Read the model definition and answer for the solid it produces. Units are mm, in the model's axes. Face numbers are marked on the shaded views. A direction names the side the tool comes from. Round coordinates to 2 decimals unless told otherwise and drop trailing zeros. Order: outer loops, then holes, each group sorted by start corner. A loop starts at its lowest first (then second) coordinate and runs counter-clockwise, first axis right, second up. Notation, with made-up numbers: (10.5, -15) -> (22.5, -15) arc R4 cw to (22.5, -8) -> close; hole circle Ø5 at (32, 24). An arc over 180 degrees is marked (long way). Use a Markdown table: item, result. Add a question column.
1. The mould has two halves that part along Z. Classify the marked faces 1, 2, 3 and 4: +Z half, -Z half, draft (parallel to the pull), parting line (faces both ways), or undercut.
2. Given pin 1 (8 mm diameter, centred on x = -3.5, z = 22, fed in from -Y), flat-ended and moving along its own axis, determine where the tip first touches the part or whether it passes through.
3. For the marked faces 5 and 6, determine the directions among +Z, -Z, +X, -X, +Y, -Y from which every point of the face is accessible in a straight line to the end or side of a thin tool.
4. Section A-A, the plane x = 0 is taken. Give the vertices of the cut face in (y, z).
5. Section B-B, the plane z = 1 is taken. Give the vertices of the cut face in (x, y), then the cut area to 3 significant figures.
6. Section C-C, the plane y = 1.75 is taken. Give the vertices of the cut face in (x, z), then the cut area to 3 significant figures.
7. Consider L1, parallel to Z at x = -0.5, y = 5.25; L2, parallel to Z at x = -10, y = -3.25; L3, parallel to X at y = -1, z = 4. Determine where each line is inside the solid, lowest interval first. Write a range as [from, to].
8. Section D-D, the plane z = 18.5 is taken. Give the vertices of the cut face in (x, y).
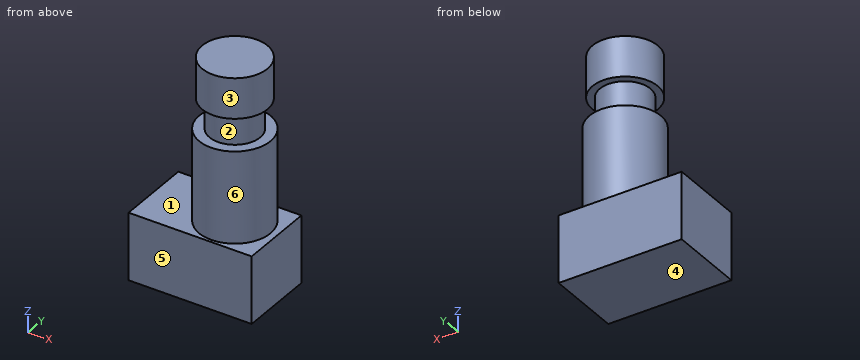
```python
from build123d import *

# Parameters (mm, degrees)
CROQUIS1_R              = 5.85
SALIENTE_EXTRUIR1_DEPTH = 15
CROQUIS2_R              = 4.15
SALIENTE_EXTRUIR2_DEPTH = 5
CROQUIS3_R              = 5.35
SALIENTE_EXTRUIR3_DEPTH = 6.6
CROQUIS4_W              = 20.15
CROQUIS4_H              = 12.4
SALIENTE_EXTRUIR4_DEPTH = 11


with BuildPart() as part:
    # Croquis1 → Saliente-Extruir1 (new body)
    with BuildSketch(Plane.XY):
        Circle(CROQUIS1_R)
    extrude(amount=SALIENTE_EXTRUIR1_DEPTH)

    # Croquis2 → Saliente-Extruir2 (add)
    with BuildSketch(Plane.XY.offset(15)):
        Circle(CROQUIS2_R)
    extrude(amount=SALIENTE_EXTRUIR2_DEPTH)

    # Croquis3 → Saliente-Extruir3 (add)
    with BuildSketch(Plane.XY.offset(20)):
        Circle(CROQUIS3_R)
    extrude(amount=SALIENTE_EXTRUIR3_DEPTH)

    # Croquis4 → Saliente-Extruir4 (add)
    with BuildSketch(Plane(origin=(0, 0, 0), x_dir=(-1, 0, 0), z_dir=(0, 0, -1))):
        with Locations((3.175, -0.113136053)):
            Rectangle(CROQUIS4_W, CROQUIS4_H)
    extrude(amount=SALIENTE_EXTRUIR4_DEPTH)


solid = part.part
```
Verdict:
| question | item | result |
|---|---|---|
| 1 | face 1 | +Z half |
| 1 | face 2 | undercut |
| 1 | face 3 | draft |
| 1 | face 4 | -Z half |
| 2 | pin 1 | stops at y = -5.35 |
| 3 | face 5 | +Z, -Z, +X, -X, -Y |
| 3 | face 6 | +Z |
| 4 | outline | (-6.31, -11) -> (6.09, -11) -> (6.09, 0) -> (5.85, 0) -> (5.85, 15) -> (4.15, 15) -> (4.15, 20) -> (5.35, 20) -> (5.35, 26.6) -> (-5.35, 26.6) -> (-5.35, 20) -> (-4.15, 20) -> (-4.15, 15) -> (-5.85, 15) -> (-5.85, 0) -> (-6.31, 0) -> close |
| 5 | outline | circle Ø11.7 at (0, 0) |
| 5 | area | 108 mm2 |
| 6 | outline | (-13.25, -11) -> (6.9, -11) -> (6.9, 0) -> (5.58, 0) -> (5.58, 15) -> (3.76, 15) -> (3.76, 20) -> (5.06, 20) -> (5.06, 26.6) -> (-5.06, 26.6) -> (-5.06, 20) -> (-3.76, 20) -> (-3.76, 15) -> (-5.58, 15) -> (-5.58, 0) -> (-13.25, 0) -> close |
| 6 | area | 493 mm2 |
| 7 | L1 | z = [-11, 15], [20, 26.6] |
| 7 | L2 | z = [-11, 0] |
| 7 | L3 | x = [-5.76, 5.76] |
| 8 | outline | circle Ø8.3 at (0, 0) |
